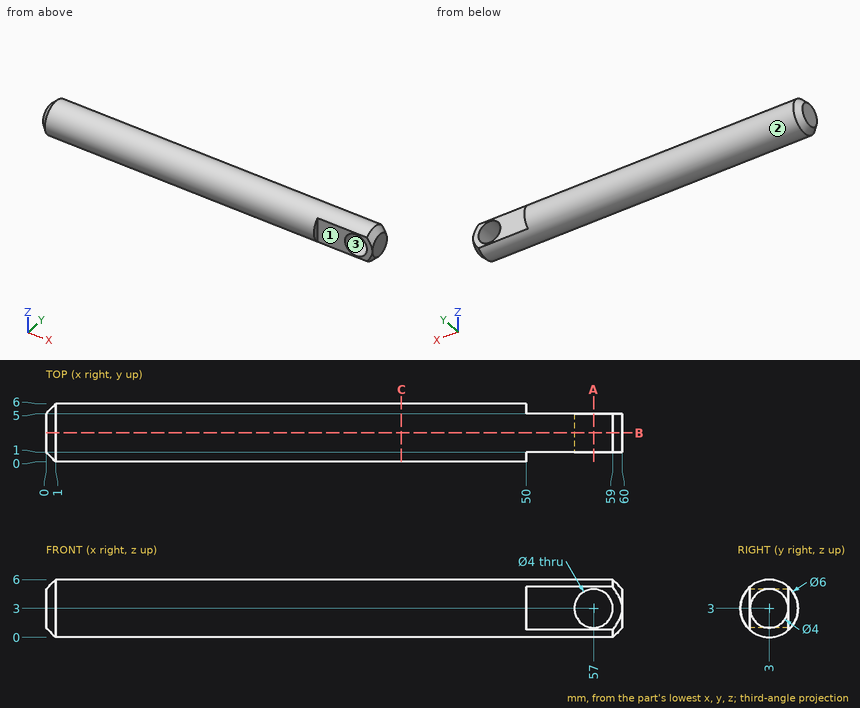
Design review of the part shown in the three views and the two pictorial views. Dimensions are in mm from the part's minimum x, y and z. Coordinates: 2 decimals unless noted, no trailing zeros. Loops run counter-clockwise (first coordinate to the right, second up) from the corner with the lowest first, then second, coordinate; pieces in that order, holes last.
Q1. We need section C-C on x = 37. State the section outline as (y, z) points.
Reported:
outline: circle Ø6 at (3, 3)
Q2. To check wall thickness, follow line 1 (Y direction, x = 51.5, z = 1.1); line 2 (Z direction, x = 57, y = 3.3); line 3 (X direction, y = 4.5, z = 3.6). State the ranges of each line that lie inside material, in increasing order.
Reported:
line 1: y = 1 to 5
line 2: z = 0.02 to 1, 5 to 5.98
line 3: x = 0 to 55.09, 58.91 to 60
Q3. The part is to be moulded in two halves that separate along Z. For the marked faces 1, 2 and 3, say which applies: +Z half, -Z half, draft (parallel to the pull), parting line (faces both ways), or undercut.
Reported:
face 1: draft
face 2: parting line
face 3: undercut
Q4. We need section B-B on y = 3. State the section outline as (x, z) points.
Reported:
outline: (0, 1) - (1, 0) - (59, 0) - (60, 1) - (60, 5) - (59, 6) - (1, 6) - (0, 5) - close; hole circle Ø4 at (57, 3)
Q5. We need section A-A on x = 57. State the section outline as (y, z) points.
Reported:
outline: (1, 0.76) arc R3 ccw to (5, 0.76) - (5, 1) - (1, 1) - close; (1, 5) - (5, 5) - (5, 5.24) arc R3 ccw to (1, 5.24) - close
Q6. For pin 1 (1 mm diameter, centred on x = 44, y = 1.5, fed in from +Z); pin 2 (3 mm diameter, centred on x = 46, y = 5, fed in from -Z); pin 3 (1 mm diameter, centred on y = 5, z = 1, fed in from -X); pin 4 (3.5 mm diameter, centred on x = 57, z = 3, fed in from -Y), all flat-tipped, find the tip position at first contact; note any pin that passes through.
Reported:
pin 1: stops at z = 5.83
pin 2: stops at z = 0.04
pin 3: stops at x = 0.33
pin 4: passes through
